Input: part model. Units: mm. Frame: model coordinates. Face numbers are marked on the shaded views. A direction names the side the tool comes from. Give positions to 0.01 mm unless a question says otherwise; leave off trailing zeros. Loops run counter-clockwise (first coordinate to the right, second up) from the corner with the lowest first, then second, coordinate; pieces in that order, holes last.
from build123d import *

# Parameters (mm, degrees)
BASE_DEPTH             = 5
SUPPORT_DEPTH          = 30
SUPPORT_DEPTH_BACK     = 30
ESQUISSE7_OUTSIDE_W    = 218.554
ESQUISSE7_OUTSIDE_H    = 101.054
AJUSTEMENT_DEPTH       = 187.832143915
TROU_CENTRE_DEPTH      = 188.500000137
ESQUISSE11_R           = 2.25
ESQUISSE11_R_2         = 5
TROU_MOTEUR_DEPTH      = 188.500000137
CONG_2_R               = 5
CONG_3_R               = 2
TROU_SUPPORT_DEPTH     = 10
ESQUISSE13_R           = 2
INSERT_HAUT_DEPTH      = 7
PONT_REACH             = 188.095
PONT_DIRECTION_2_DEPTH = 187.094734075
ESQUISSE14_R           = 2
INSERT_BAS_DEPTH       = 7


with BuildPart() as part:
    # Esquisse2 → Base (new body)
    with BuildSketch(Plane(origin=(0, 0, 0), x_dir=(1, 0, 0), z_dir=(0, 1, 0))):
        with BuildLine():
            ThreePointArc((-10, 25), (-82.734029234, 15.101895807), (-156.112273553, 17.062695657))
            ThreePointArc((-156.112273553, 17.062695657), (-177.5, 0), (-156.112273553, -17.062695657))
            ThreePointArc((-156.112273553, -17.062695657), (-82.734029234, -15.101895807), (-10, -25))
            Line((-10, -25), (0, -25))
            Line((0, -25), (0, 25))
            Line((0, 25), (-10, 25))
        make_face()
    extrude(amount=BASE_DEPTH)

    # Esquisse6 → Support (add, two sides: drawn at the far end of the back side and taken through both)
    with BuildSketch(Plane.XY.offset(-SUPPORT_DEPTH_BACK)):
        with BuildLine():
            Line((0, 0), (0, -50))
            Line((0, -50), (-15, -50))
            ThreePointArc((-15, -50), (-92.49080932, -12.782630291), (-177.5, 0))
            Line((-177.5, 0), (-111.226419291, 0))
            ThreePointArc((-111.226419291, 0), (-61.29219157, -16.216276522), (-15, -40.983749587))
            Line((-15, -40.983749587), (-15, 0))
            Line((-15, 0), (0, 0))
        make_face()
    extrude(amount=SUPPORT_DEPTH + SUPPORT_DEPTH_BACK)

    # Esquisse7 outside → Ajustement (cut, through all)
    with BuildSketch(Plane(origin=(0, 0, 0), x_dir=(1, 0, 0), z_dir=(0, 1, 0))):
        with Locations((-88.75, 0)):
            Rectangle(ESQUISSE7_OUTSIDE_W, ESQUISSE7_OUTSIDE_H)
        with BuildLine():
            Line((-10, -25), (0, -25))
            Line((0, -25), (0, 25))
            Line((0, 25), (-10, 25))
            ThreePointArc((-10, 25), (-82.734029234, 15.101895807), (-156.112273553, 17.062695657))
            ThreePointArc((-156.112273553, 17.062695657), (-177.5, 0), (-156.112273553, -17.062695657))
            ThreePointArc((-156.112273553, -17.062695657), (-82.734029234, -15.101895807), (-10, -25))
        make_face(mode=Mode.SUBTRACT)
    extrude(amount=-AJUSTEMENT_DEPTH, mode=Mode.SUBTRACT)

    # Esquisse9 → Trou_centre (cut, through all)
    with BuildSketch(Plane(origin=(0, 5, 0), x_dir=(1, 0, 0), z_dir=(0, 1, 0))):
        with BuildLine():
            Line((-15, -13.722068475), (-15, 13.722068475))
            ThreePointArc((-15, 13.722068475), (-78.978011617, 5.302380383), (-143.505381198, 5.846156906))
            ThreePointArc((-143.505381198, 5.846156906), (-142.5, 0), (-143.505381198, -5.846156906))
            ThreePointArc((-143.505381198, -5.846156906), (-78.978011617, -5.302380383), (-15, -13.722068475))
        make_face()
    extrude(amount=-TROU_CENTRE_DEPTH, mode=Mode.SUBTRACT)

    # Esquisse11 → Trou_moteur (cut, through all)
    with BuildSketch(Plane(origin=(0, 5, 0), x_dir=(1, 0, 0), z_dir=(0, 1, 0))):
        with Locations(Location((-153.282485579, 6.717514421, 0), (0, 0, 270))):
            Circle(ESQUISSE11_R)
        with Locations(Location((-153.282485579, -6.717514421, 0), (0, 0, 270))):
            Circle(ESQUISSE11_R)
        with Locations(Location((-166.717514421, -6.717514421, 0), (0, 0, 270))):
            Circle(ESQUISSE11_R)
        with Locations(Location((-166.717514421, 6.717514421, 0), (0, 0, 270))):
            Circle(ESQUISSE11_R)
        with Locations(Location((-160, 0, 0), (0, 0, 270))):
            Circle(ESQUISSE11_R_2)
    extrude(amount=-TROU_MOTEUR_DEPTH, mode=Mode.SUBTRACT)

    # Congé2
    cong_2_edges = [part.edges().sort_by_distance(p)[0] for p in [
        (-15, -40.983749587, 18.826594184),
        (-15, -40.983749587, -18.826594184),
        (-15, 0, -18.826594184),
        (-15, 0, 18.826594184),
    ]]
    fillet(cong_2_edges, radius=CONG_2_R)

    # Congé3
    cong_3_edges = [part.edges().sort_by_distance(p)[0] for p in [
        (-111.226419291, 0, -9.45038232),
        (-111.226419291, 0, 9.45038232),
    ]]
    fillet(cong_3_edges, radius=CONG_3_R)

    # Esquisse12 → Trou_support (cut)
    with BuildSketch(Plane(origin=(0, 5, 0), x_dir=(1, 0, 0), z_dir=(0, 1, 0))):
        Polygon((-15, -5.1), (-10, -5.1), (-10, -25), (0, -25), (0, 25), (-10, 25), (-10, 5.1), (-15, 5.1), align=None)
    extrude(amount=-TROU_SUPPORT_DEPTH, mode=Mode.SUBTRACT)

    # Esquisse13 → Insert_haut (cut)
    with BuildSketch(Plane(origin=(0, -5, 0), x_dir=(1, 0, 0), z_dir=(0, 1, 0))):
        with Locations(Location((-5, -15.1, 0), (0, 0, 270))):
            Circle(ESQUISSE13_R)
        with Locations(Location((-5, 15.1, 0), (0, 0, 270))):
            Circle(ESQUISSE13_R)
    extrude(amount=-INSERT_HAUT_DEPTH, mode=Mode.SUBTRACT)

    # Esquisse15 → Pont (cut, up to next)
    with BuildSketch(Plane(origin=(0, 0, 0), x_dir=(0, 0, -1), z_dir=(1, 0, 0)), mode=Mode.PRIVATE) as pont_sk1:
        with BuildLine():
            Line((-9, -50), (-9, -30))
            ThreePointArc((-9, -30), (0, -21), (9, -30))
            Line((9, -30), (9, -50))
            Line((9, -50), (-9, -50))
        make_face()
    pont_tool1 = extrude(pont_sk1.sketch, amount=-PONT_REACH, mode=Mode.PRIVATE) & part.part
    add(pont_tool1.solids().sort_by_distance((0, -36.391173, 0))[0], mode=Mode.SUBTRACT)

    # Esquisse15 → Pont direction 2 (cut)
    with BuildSketch(Plane(origin=(0, 0, 0), x_dir=(0, 0, -1), z_dir=(1, 0, 0))):
        with BuildLine():
            Line((-9, -50), (-9, -30))
            ThreePointArc((-9, -30), (0, -21), (9, -30))
            Line((9, -30), (9, -50))
            Line((9, -50), (-9, -50))
        make_face()
    extrude(amount=PONT_DIRECTION_2_DEPTH, mode=Mode.SUBTRACT)

    # Esquisse14 → Insert_bas (cut)
    with BuildSketch(Plane.XZ.offset(50)):
        with Locations(Location((-7.5, 17, 0), (0, 0, 270))):
            Circle(ESQUISSE14_R)
        with Locations(Location((-7.5, -17, 0), (0, 0, 270))):
            Circle(ESQUISSE14_R)
    extrude(amount=-INSERT_BAS_DEPTH, mode=Mode.SUBTRACT)


solid = part.part
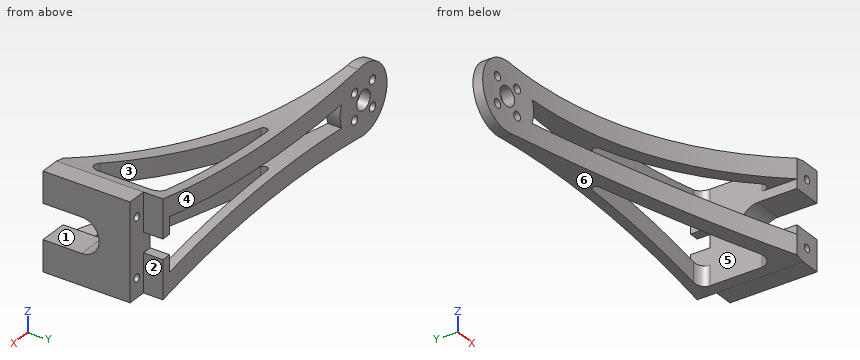
(1) Ray query, probe 1 along Z at (x, y) = (-7, -47); probe 2 along Y at (x, z) = (-57, 15.5); probe 3 along Y at (x, z) = (-74, 10.5). Return the intervals inside material, ascending.
Values follow:
probe 1: z = -25 to -18.94, -15.06 to -9, 9 to 15.06, 18.94 to 25
probe 2: y = -26.31 to -18.08, 0 to 5
probe 3: y = -19.16 to -11.15, 0 to 5
(2) Cut plane A-A (x = -39). Return the cut outline in (y, z).
Values follow:
outline: (-35.34, -19.61) - (-26.83, -19.61) - (-26.83, -9.5) - (-35.34, -9.5) - close; (-35.34, 9.5) - (-26.83, 9.5) - (-26.83, 19.61) - (-35.34, 19.61) - close; (0, -19.61) - (5, -19.61) - (5, -9.5) - (0, -9.5) - close; (0, 9.5) - (5, 9.5) - (5, 19.61) - (0, 19.61) - close
(3) Cut plane D-D (x = -82). Return the cut outline in (y, z).
Values follow:
outline: (-16.23, -15.14) - (-8.3, -15.14) - (-8.3, -5.13) - (-16.23, -5.13) - close; (-16.23, 5.13) - (-8.3, 5.13) - (-8.3, 15.14) - (-16.23, 15.14) - close; (0, -15.14) - (5, -15.14) - (5, -5.13) - (0, -5.13) - close; (0, 5.13) - (5, 5.13) - (5, 15.14) - (0, 15.14) - close
(4) Cut plane B-B (z = 0). Return the cut outline in (x, y) (1 decimal).
Values follow:
outline: (-177.5, 0) arc R289.1 cw to (-165, -0.3) - (-165, 5) - (-177.5, 5) - close; (-155, -0.9) arc R289.1 cw to (-142.5, -2.1) - (-142.5, 5) - (-155, 5) - close; (-15, -21) - (0, -21) - (0, -5) - (-15, -5) - close
(5) Reachability of the marked faces 1, 2 and 3 from +Z, -Z, +X, -X, +Y, -Y: full face, straight path, thin tool, end or side. Return the list, or none.
Values follow:
face 1: +X, -Y
face 2: +Z, -Z, +X, +Y
face 3: +Z, -Z
(6) Pin query (flat end, axial travel): pin 1 Ø5 at (x, z) = (-80, 19) entering from +Y; pin 2 Ø4.5 at (x, z) = (-5, -14) entering from +Y; pin 3 Ø7 at (x, z) = (-153.28, 6.72) entering from -Y; pin 4 Ø9 at (x, z) = (-72.5, -13.5) entering from -Y. Return the tip coordinate at first contact, or that it passes through.
Values follow:
pin 1: passes through
pin 2: stops at y = -5
pin 3: stops at y = -1.33
pin 4: stops at y = -21.54
(7) Mould query, pull axis Z, two halves, no side actions, for the marked faces 4, 5 and 6. Classes: +Z half, -Z half, draft (parallel to the pull), parting line (faces both ways), or undercut.
Values follow:
face 4: draft
face 5: undercut
face 6: -Z half
(8) Cut plane C-C (x = -119.5). Return the cut outline in (y, z), and give its area (3 significant figures).
Values follow:
outline: (-5.88, -14.6) - (5, -14.6) - (5, -4.59) - (-5.88, -4.59) - close; (-5.88, 4.59) - (5, 4.59) - (5, 14.6) - (-5.88, 14.6) - close
area: 218 mm2
